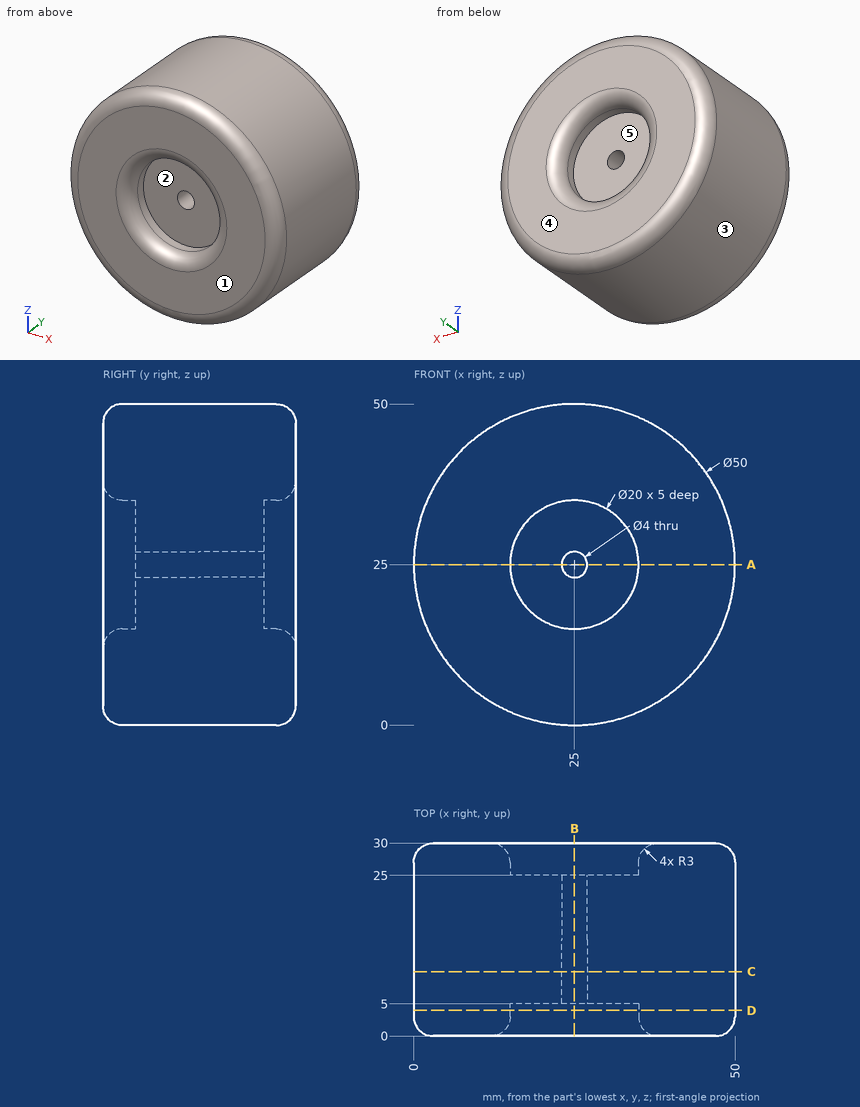
For this review, use the dimensioned drawing (mm, ordinates from the lowest corner) and the shaded views. A direction names the side the tool comes from. Give positions to 0.01 mm unless a question says otherwise; leave off trailing zeros. Loops run counter-clockwise (first coordinate to the right, second up) from the corner with the lowest first, then second, coordinate; pieces in that order, holes last. Notation, with made-up numbers: (67.5, 29) -> (98.5, 29) arc R9 ccw to (98.5, 37) -> close; hole circle Ø10 at (-9.75, -23). An arc over 180 degrees is marked (long way). One line per question, with ' | ' between items. Start each with the question number.
(1) For the marked faces 1 and 2, list the 3-axis set-ups (+Z, -Z, +X, -X, +Y, -Y) from which the entire face can be reached by the end or side of a thin tool; tool diameter is ignored.
(2) We need section B-B (x = 25). State the section outline as (y, z) points, and give its area (3 significant figures).
(3) We need section A-A (z = 25). State the section outline as (x, y) points, and give its area (3 significant figures).
(4) Insertion check: P1, Ø4.5, axis at x = 25, z = 25, coming from the +Y side; P2, Ø5, axis at x = 7, z = 7.5, coming from the +Y side; P3, Ø5, axis at x = 6, y = 13.5, coming from the -Z side. Each pin has a flat end and moves straight along its axis. Give the tip position at first contact, or say it passes through.
(5) Draft analysis for pull direction Z (two halves, no side actions). For the marked faces 3, 4 and 5, state which applies: +Z half, -Z half, draft (parallel to the pull), parting line (faces both ways), or undercut.
(6) We need section C-C (y = 10). State the section outline as (x, z) points, and give its area (3 significant figures).
(7) We need section D-D (y = 4). State the section outline as (x, z) points.
(8) For line 1 (Z direction, x = 25, y = 20.25); line 2 (X direction, y = 28.5, z = 26); line 3 (Y direction, x = 25, z = 31.5), list the stretches that pass through material, from the lowest coordinate up.
The answers:
1) face 1: +Z, -Z, +X, -X, -Y | face 2: -Y
2) outline: (0, 3) arc R3 ccw to (3, 0) -> (27, 0) arc R3 ccw to (30, 3) -> (30, 12) arc R3 ccw to (27, 15) -> (25, 15) -> (25, 23) -> (5, 23) -> (5, 15) -> (3, 15) arc R3 ccw to (0, 12) -> close; (0, 38) arc R3 ccw to (3, 35) -> (5, 35) -> (5, 27) -> (25, 27) -> (25, 35) -> (27, 35) arc R3 ccw to (30, 38) -> (30, 47) arc R3 ccw to (27, 50) -> (3, 50) arc R3 ccw to (0, 47) -> close | area: 1,200 mm^2
3) outline: (0, 3) arc R3 ccw to (3, 0) -> (12, 0) arc R3 ccw to (15, 3) -> (15, 5) -> (23, 5) -> (23, 25) -> (15, 25) -> (15, 27) arc R3 ccw to (12, 30) -> (3, 30) arc R3 ccw to (0, 27) -> close; (27, 5) -> (35, 5) -> (35, 3) arc R3 ccw to (38, 0) -> (47, 0) arc R3 ccw to (50, 3) -> (50, 27) arc R3 ccw to (47, 30) -> (38, 30) arc R3 ccw to (35, 27) -> (35, 25) -> (27, 25) -> close | area: 1,200 mm^2
4) P1: stops at y = 25 | P2: stops at y = 29.94 | P3: stops at z = 6.22
5) face 3: parting line | face 4: draft | face 5: undercut
6) outline: circle Ø50 at (25, 25); hole circle Ø4 at (25, 25) | area: 1,950 mm^2
7) outline: circle Ø50 at (25, 25); hole circle Ø20 at (25, 25)
8) line 1: z = 0 to 23, 27 to 50 | line 2: x = 0.42 to 14.65, 35.35 to 49.58 | line 3: y = 5 to 25
